Can you work these out from the model? Positions are in its coordinate system, mm. A direction names the side the tool comes from. Give positions to 0.01 mm unless a question says otherwise; leave off trailing zeros. Write each loop counter-clockwise with the first axis right and the second up, starting at its lowest first coordinate (ties: lowest second). Pieces come first, ordered by that corner, then holes.
```python
from build123d import *

# Parameters (mm, degrees)
SKETCH_2_R          = 4
CUT_EXTRUDE_1_DEPTH = 20.595917942


with BuildPart() as part:
    # 草图1 → 旋转1 (revolve)
    with BuildSketch(Plane.XY, mode=Mode.PRIVATE) as revolve_1_sk:
        Polygon((0, 14.15), (-8, 14.15), (-8, 13.15), (-6, 13.15), (-6, 6.15), (-8, 6.15), (-8, -1.85), (0, -1.85), align=None)
    revolve(revolve_1_sk.sketch.rotate(Axis((0, 15.9, 0), (0, -1, 0)), 270), axis=Axis((0, 15.9, 0), (0, -1, 0)))

    # 草图2 → 切除-拉伸1 (cut, through all)
    with BuildSketch(Plane.XZ.offset(1.85)):
        with Locations(Location((0, 0, 0), (0, 0, 270))):
            Circle(SKETCH_2_R)
    extrude(amount=-CUT_EXTRUDE_1_DEPTH, mode=Mode.SUBTRACT)


solid = part.part
```
1) For pin 1 Ø8 at (y, z) = (9.5, 4.5) entering from +X; pin 2 Ø8 at (y, z) = (10, 4) entering from -X; pin 3 Ø1 at (y, z) = (4, 5) entering from +X; pin 4 Ø5 at (x, z) = (-1, 1) entering from +Y (1 decimal), each with a flat end and sliding along its axis, tell me the tip position at first contact or that it passes through.
Values follow:
pin 1: stops at x = 7.66
pin 2: stops at x = -7.85
pin 3: stops at x = 6.61
pin 4: passes through
2) Suppose I cut it at B-B on z = 3.5. Write out the boundary of the cut face in (x, y).
Values follow:
outline: (-7.19, -1.85) - (-1.94, -1.85) - (-1.94, 14.15) - (-7.19, 14.15) - (-7.19, 13.15) - (-4.87, 13.15) - (-4.87, 6.15) - (-7.19, 6.15) - close; (1.94, -1.85) - (7.19, -1.85) - (7.19, 6.15) - (4.87, 6.15) - (4.87, 13.15) - (7.19, 13.15) - (7.19, 14.15) - (1.94, 14.15) - close
3) Suppose I cut it at D-D on x = -5. Write out the boundary of the cut face in (y, z) (3 decimals), plus the area to 3 significant figures.
Values follow:
outline: (-1.85, -6.245) - (6.15, -6.245) - (6.15, -3.317) - (13.15, -3.317) - (13.15, -6.245) - (14.15, -6.245) - (14.15, 6.245) - (13.15, 6.245) - (13.15, 3.317) - (6.15, 3.317) - (6.15, 6.245) - (-1.85, 6.245) - close
area: 159 mm2
4) If we mould it in two halves opening along Y, with no side actions, what happens to faces 3 (the face through (-6, 13.15, -2)), 4 (the face through (2, 14.15, 4)), 5 (the face through (-3.905, 6.038, 0.867))? For each: +Y half, -Y half, draft (parallel to the pull), parting line (faces both ways), or undercut.
Values follow:
face 3: undercut
face 4: +Y half
face 5: draft
5) For faces 1 (the face through (2, -1.85, -4)), 2 (the face through (-6, 6.15, 2)), which set-ups out of +Z, -Z, +X, -X, +Y, -Y let a thin tool reach every point of the face, with its end or its side?
Values follow:
face 1: +Z, -Z, +X, -X, -Y
face 2: none
6) Suppose I cut it at A-A on x = 0. Write out the boundary of the cut face in (y, z).
Values follow:
outline: (-1.85, -8) - (6.15, -8) - (6.15, -6) - (13.15, -6) - (13.15, -8) - (14.15, -8) - (14.15, -4) - (-1.85, -4) - close; (-1.85, 4) - (14.15, 4) - (14.15, 8) - (13.15, 8) - (13.15, 6) - (6.15, 6) - (6.15, 8) - (-1.85, 8) - close
7) Suppose I cut it at C-C on y = 1. Write out the boundary of the cut face in (x, z), plus the area to 3 significant figures.
Values follow:
outline: circle Ø16 at (0, 0); hole circle Ø8 at (0, 0)
area: 151 mm2
8) Please list where these lines run through material, in increasing order: L1, parallel to Y at x = 4.25, z = 5.5; L2, parallel to X at y = 7.25, z = 0; L3, parallel to X at y = 3.75, z = 0.
Values follow:
L1: y = -1.85 to 6.15, 13.15 to 14.15
L2: x = -6 to -4, 4 to 6
L3: x = -8 to -4, 4 to 8
